from build123d import *

# Parameters (mm, degrees)
SKETCH1_R           = 21.5
BOSS_EXTRUDE1_DEPTH = 4
SKETCH2_R           = 21.5
SKETCH2_R_2         = 13.5
BOSS_EXTRUDE2_DEPTH = 50
SKETCH3_R           = 2
CUT_EXTRUDE1_DEPTH  = 6
CIRPATTERN1_COUNT   = 3
CUT_EXTRUDE2_REACH  = 63.972
SKETCH4_W           = 3
SKETCH4_H           = 3


with BuildPart() as part:
    # Sketch1 → Boss-Extrude1 (new body)
    with BuildSketch(Plane(origin=(0, 0, 0), x_dir=(1, 0, 0), z_dir=(0, 1, 0))):
        with Locations(Location((0, 0, 0), (0, 0, 270))):
            Circle(SKETCH1_R)
    extrude(amount=BOSS_EXTRUDE1_DEPTH)

    # Sketch2 → Boss-Extrude2 (add)
    with BuildSketch(Plane(origin=(0, 4, 0), x_dir=(1, 0, 0), z_dir=(0, 1, 0))):
        with Locations(Location((0, 0, 0), (0, 0, 270))):
            Circle(SKETCH2_R)
        with Locations(Location((0, 0, 0), (0, 0, 270))):
            Circle(SKETCH2_R_2, mode=Mode.SUBTRACT)
    extrude(amount=BOSS_EXTRUDE2_DEPTH)

    # Sketch3 → Cut-Extrude1 (cut)
    with BuildSketch(Plane(origin=(0, 54, 0), x_dir=(1, 0, 0), z_dir=(0, 1, 0))):
        with Locations(Location((0, 17.5, 0), (0, 0, 270))):
            Circle(SKETCH3_R)
    cut_extrude1 = extrude(amount=-CUT_EXTRUDE1_DEPTH, mode=Mode.SUBTRACT)

    # CirPattern1: Cut-Extrude1 ×3 about axis
    cirpattern1_axis = Axis((0, 0, 0), (0, 1, 0))
    for i in range(1, CIRPATTERN1_COUNT):
        add(cut_extrude1.rotate(cirpattern1_axis, i * 360 / CIRPATTERN1_COUNT), mode=Mode.SUBTRACT)

    # Sketch4 → Cut-Extrude2 (cut, up to next)
    with BuildSketch(Plane.XZ, mode=Mode.PRIVATE) as cut_extrude2_sk1:
        Rectangle(SKETCH4_W, SKETCH4_H)
    cut_extrude2_tool1 = extrude(cut_extrude2_sk1.sketch, amount=-CUT_EXTRUDE2_REACH, mode=Mode.PRIVATE) & part.part
    add(cut_extrude2_tool1.solids().sort_by_distance((0, 0, 0))[0], mode=Mode.SUBTRACT)


solid = part.part
Geometry check sheet. Reference: the model listing, model coordinates, mm. A direction names the side the tool comes from. Round coordinates to 2 decimals unless told otherwise and drop trailing zeros. Loops run counter-clockwise (first coordinate to the right, second up) from the corner with the lowest first, then second, coordinate; pieces in that order, holes last. Notation, with made-up numbers: (-35, -37) -> (-6, -37) arc R25 ccw to (-6, -18) -> close; hole circle Ø2 at (-13, 76). An arc over 180 degrees is marked (long way). Answer as a JSON object with one key per item and string values. Group by question number.
Item 1: Set-up check for faces 1 (the face through (15, 48, 9)), 2 (the face through (0, 0, 4)), 3 (the face through (0, 2, 1.5)): record each of +Z, -Z, +X, -X, +Y, -Y from which the full face is reachable in a straight line by a thin tool's end or side.
Item 2: Cross-section at A-A, the plane z = 0. Record the cut outline in (x, y), plus the area to 3 significant figures.
Item 3: Depth check by flat-ended pin: pin 1 Ø1.2 at (x, z) = (-15, 8.5) entering from +Y; pin 2 Ø4 at (y, z) = (47, 2.5) entering from +X; pin 3 Ø3 at (y, z) = (12, -12.5) entering from -X. Enter the tip coordinate at first touch or a pass-through.
Item 4: Release check for a two-part mould opening along Z. For faces 4 (the face through (-14, 54, 0)), 5 (the face through (14.531, 26.622, -15.846)), 6 (the face through (0, 48, -18)) record: pulls with the +Z half, pulls with the -Z half, needs draft (parallel to the pull), parting line crosses it, or undercut.
Item 5: Cross-section at D-D, the plane z = -17.5. Record the cut outline in (x, y), plus the area to 3 significant figures.
Item 6: Thickness scan on line 1 along X through (y, z) = (49.8, 8.75); line 2 along X through (y, z) = (52, 8); line 3 along X through (y, z) = (36.5, 0). Record the ranges inside material, lowest first.
Item 7: Cross-section at C-C, the plane y = 26.5. Record the cut outline in (x, z), plus the area to 3 significant figures.
Item 8: Cross-section at B-B, the plane x = 0. Record the cut outline in (y, z).
Determined:
{
 "1": {"face 1": "+Y", "face 2": "+Z, -Z, +X, -X, -Y", "face 3": "+Y, -Y"},
 "2": {"outline": "(-21.5, 0) -> (-1.5, 0) -> (-1.5, 4) -> (-13.5, 4) -> (-13.5, 54) -> (-21.5, 54) -> close; (1.5, 0) -> (21.5, 0) -> (21.5, 54) -> (13.5, 54) -> (13.5, 4) -> (1.5, 4) -> close", "area": "960 mm²"},
 "3": {"pin 1": "stops at y = 48", "pin 2": "stops at x = 21.49", "pin 3": "stops at x = -18.47"},
 "4": {"face 4": "needs draft", "face 5": "parting line crosses it", "face 6": "undercut"},
 "5": {"outline": "(-12.49, 0) -> (12.49, 0) -> (12.49, 54) -> (2, 54) -> (2, 48) -> (-2, 48) -> (-2, 54) -> (-12.49, 54) -> close", "area": "1,320 mm²"},
 "6": {"line 1": "x = -19.64 to -17.16, -13.16 to -10.28, 10.28 to 13.16, 17.16 to 19.64", "line 2": "x = -19.96 to -17.01, -13.3 to -10.87, 10.87 to 13.3, 17.01 to 19.96", "line 3": "x = -21.5 to -13.5, 13.5 to 21.5"},
 "7": {"outline": "circle Ø43 at (0, 0); hole circle Ø27 at (0, 0)", "area": "880 mm²"},
 "8": {"outline": "(0, -21.5) -> (54, -21.5) -> (54, -19.5) -> (48, -19.5) -> (48, -15.5) -> (54, -15.5) -> (54, -13.5) -> (4, -13.5) -> (4, -1.5) -> (0, -1.5) -> close; (0, 1.5) -> (4, 1.5) -> (4, 13.5) -> (54, 13.5) -> (54, 21.5) -> (0, 21.5) -> close"}
}
